Autodesk Inventor part; units mm, degrees
sketch "Skizze1" plane through (0, 0, 0) normal (0, 0, 1) x (1, 0, 0)
  line L0 (0, 40) -> (0, -37) construction
  line L1 (-52, 0) -> (54, 0) construction
  line L2 (-90, -55) -> (90, -55)
  line L3 (90, -55) -> (90, 55)
  line L4 (90, 55) -> (-90, 55)
  line L5 (-90, 55) -> (-90, -55)
  line L6 (0, -77) -> (0, 77)
  line L7 (-126, 0) -> (126, 0)
  point P0 (0, 0)
  dimension "d0" = 110
  dimension "d1" = 180
extrude "Extrusion1" add sketch "Skizze1" along normal blind 8
sketch "Skizze2" plane through (0, 0, 8) normal (0, 0, 1) x (1, 0, 0)
  line L0 (-75, 40) -> (-15, 40)
  line L1 (-15, 40) -> (-15, -40)
  line L2 (-15, -40) -> (-75, -40)
  line L3 (-75, -40) -> (-75, 40)
  line L4 (-126, 0) -> (126, 0)
  line L5 (0, 77) -> (0, -77)
  point P0 (0, 0)
  dimension "d4" = 60
  dimension "d5" = 80
  dimension "d6" = 15
extrude "Extrusion2" cut sketch "Skizze2" against normal blind 7
sketch "Skizze3" plane through (0, 0, 1) normal (0, 0, 1) x (1, 0, 0)
  line L0 (-15, 40) -> (-15, -40)
  line L1 (-15, -40) -> (-75, -40)
  line L2 (-75, -40) -> (-75, 40)
  line L3 (-15, -40) -> (-75, -40)
  line L4 (-15, 40) -> (-15, -40)
  line L5 (-75, 40) -> (-15, 40)
  line L6 (-126, 0) -> (126, 0)
  line L7 (0, 77) -> (0, -77)
  circle A0 centre (-45, -25) radius 4
  point P0 (0, 0)
  dimension "d9" = 8
  dimension "d10" = 30
  dimension "d11" = 15
extrude "Extrusion3" cut sketch "Skizze3" against normal blind 10 contours A0
sketch "Skizze4" plane through (0, 0, 1) normal (0, 0, 1) x (1, 0, 0)
  circle A0 centre (-45, -25) radius 4
  line L0 (-75, -40) -> (-75, 40)
  line L1 (-15, -40) -> (-75, -40)
  line L2 (-15, 40) -> (-15, -40)
  line L3 (-75, 40) -> (-15, 40)
  line L4 (-126, 0) -> (126, 0)
  line L5 (-67, 27.5) -> (-62, 27.5)
  line L6 (-62, 27.5) -> (-62, -27.5)
  line L7 (-62, -27.5) -> (-67, -27.5)
  line L8 (-67, -27.5) -> (-67, 27.5)
  line L9 (-23, 27.5) -> (-28, 27.5)
  line L10 (-28, 27.5) -> (-28, -27.5)
  line L11 (-28, -27.5) -> (-23, -27.5)
  line L12 (-23, -27.5) -> (-23, 27.5)
  point P0 (0, 0)
  dimension "d14" = 5
  dimension "d15" = 55
  dimension "d16" = 8
  dimension "d17" = 55
  dimension "d18" = 5
  dimension "d19" = 8
extrude "Extrusion4" add sketch "Skizze4" along normal blind 5.5 contours L8 L5 L6 L4 | L4 L6 L7 L8 | L12 L11 L10 L4 | L4 L10 L9 L12
sketch "Skizze5" plane through (0, 0, 8) normal (0, 0, 1) x (1, 0, 0)
  line L0 (0, 77) -> (0, -77)
  line L1 (-126, 0) -> (126, 0)
  circle A0 centre (0, 30) radius 3
  circle A1 centre (0, -30) radius 3
  point P0 (0, 0)
  dimension "d22" = 6
  dimension "d23" = 6
  dimension "d24" = 30
  dimension "d25" = 30
extrude "Extrusion5" cut sketch "Skizze5" against normal blind 10
sketch "Skizze6" plane through (0, 0, 8) normal (0, 0, 1) x (1, 0, 0)
  line L0 (-75, 40) -> (-15, 40)
  line L1 (-75, -40) -> (-75, 40)
  line L2 (-67, 27.5) -> (-67, -27.5)
  line L3 (-62, -27.5) -> (-62, 27.5)
  line L4 (-62, 27.5) -> (-67, 27.5)
  line L5 (-67, -27.5) -> (-62, -27.5)
  line L6 (-15, -40) -> (-75, -40)
  circle A0 centre (-45, -25) radius 4
  line L7 (-28, 27.5) -> (-28, -27.5)
  line L8 (-28, -27.5) -> (-23, -27.5)
  line L9 (-23, -27.5) -> (-23, 27.5)
  line L10 (-23, 27.5) -> (-28, 27.5)
  line L11 (-28, 27.5) -> (-28, -27.5)
  line L12 (-28, -27.5) -> (-23, -27.5)
  line L13 (-15, 40) -> (-15, -40)
  line L14 (0, 77) -> (0, -77)
  line L15 (-126, 0) -> (126, 0)
  point P0 (0, 0)
mirror "Spiegeln1" about plane through (0, 0, 0) normal (1, 0, 0) of "Extrusion4", "Extrusion2", "Extrusion3"
sketch "Skizze7" plane through (0, 0, 0) normal (0, 0, -1) x (-1, 0, 0)
  point P0 (0, 0)
sketch "Skizze8" plane through (0, 0, 0) normal (1, 0, 0) x (0, 1, 0)
  circle A0 centre (0, -7) radius 1.65
  circle A1 centre (0, -7) radius 4
  line L0 (55, 0) -> (-55, 0)
  line L1 (4, 0) -> (4, -7)
  line L2 (-4, -7) -> (-4, 0)
  point P0 (0, 0)
  dimension "d28" = 3.3
  dimension "d29" = 7
  dimension "d30" = 8
extrude "Extrusion6" add sketch "Skizze8" along normal mid plane 6
pattern_linear "Rechteckige Anordnung1" count 2 spacing 80 along (-1, 0, 0) of "Extrusion6"
pattern_linear "Rechteckige Anordnung2" count 2 spacing 80 along (1, 0, 0) of "Extrusion6"
chamfer "Fase1" distance 6 angle 45 4 edges at (0, 55, 8) (-90, 0, 8) (0, -55, 8) (90, 0, 8)
properties part number "PV-Halterung"
Source: CAD feature listing. Evaluate the final solid. Frame: model axes, mm. A direction names the side the tool comes from. Give positions to 0.01 mm unless a question says otherwise; leave off trailing zeros. Order: outer loops, then holes, each group sorted by start corner. A loop starts at its lowest first (then second) coordinate and runs counter-clockwise, first axis right, second up.
(1) Pull-direction query (Y, two-part tool) for faces 1 (the face through (-28, 0, 4)), 2 (the face through (0, -4, -4)), 3 (the face through (45, 1, 1)), 4 (the face through (-1, 13, 0)); classes: +Y half, -Y half, draft (parallel to the pull), parting line (faces both ways), or undercut.
(2) Section query A-A (y = 30). Return the cut outline in (x, z), plus the area to 3 significant figures.
(3) Contact query for flat-ended pins moving along their axis: P1, Ø8, axis at y = 8, z = 5, coming from the -X side; P2, Ø6, axis at y = 6.5, z = -7.5, coming from the +X side; P3, Ø1.8, axis at x = 81, z = -4, coming from the +Y side; P4, Ø4, axis at y = 0, z = -7.5, coming from the -X side. Output: stop coordinate, or through.
(4) Section query C-C (x = 45). Return the cut outline in (y, z).
(5) Section query D-D (y = -25). State how many separate pieces and enclosed holes the cut face has, plus the area to 3 significant figures.
(6) Material intervals for line 1 along Y through (x, z) = (-31, 2); line 2 along Y through (x, z) = (45, 0.7); line 3 along Y through (x, z) = (-27, 5.75), sorted ascending.
(7) Access query for faces 5 (the face through (83, 0, -4)), 6 (the face through (-83, 0, -4)), 7 (the face through (-3, 0, -4)), 8 (the face through (80, -4, -4)), 9 (the face through (-67, 0, 4)). Directions: +Z, -Z, +X, -X, +Y, -Y. A direction counts if a zero-diameter tool reaches every point of the face in a straight line with its end or side. Return the directions, or none.
(8) Section query B-B (z = -2.75). Return the cut outline in (x, y).
Outcome:
1. face 1: undercut
1. face 2: -Y half
1. face 3: undercut
1. face 4: draft
2. outline: (-90, 0) - (-3, 0) - (-3, 8) - (-15, 8) - (-15, 1) - (-75, 1) - (-75, 8) - (-84, 8) - (-90, 2) - close; (3, 0) - (90, 0) - (90, 2) - (84, 8) - (75, 8) - (75, 1) - (15, 1) - (15, 8) - (3, 8) - close
2. area: 516 mm2
3. P1: stops at x = -90
3. P2: stops at x = 83
3. P3: stops at y = 4
3. P4: stops at x = -83
4. outline: (-55, 0) - (-29, 0) - (-29, 1) - (-40, 1) - (-40, 8) - (-49, 8) - (-55, 2) - close; (-21, 0) - (55, 0) - (55, 2) - (49, 8) - (40, 8) - (40, 1) - (-21, 1) - close
5. separate pieces: 3
5. enclosed holes: 0
5. area: 658 mm2
6. line 1: y = -55 to -40, 40 to 55
6. line 2: y = -55 to -29, -21 to 55
6. line 3: y = -51.25 to -40, -27.5 to 27.5, 40 to 51.25
7. face 5: -Z, +X, +Y, -Y
7. face 6: -Z, -X, +Y, -Y
7. face 7: -Z, +Y, -Y
7. face 8: -Z, +X, -X, -Y
7. face 9: +Z
8. outline: (-83, -4) - (-77, -4) - (-77, 4) - (-83, 4) - close; (-3, -4) - (3, -4) - (3, 4) - (-3, 4) - close; (77, -4) - (83, -4) - (83, 4) - (77, 4) - close
